```python
from build123d import *

# Parameters (mm, degrees)
F0_R          = 12.7
F1_DEPTH      = 7.874
F3_DEPTH      = 25.4
F3_DEPTH_BACK = 25.4
F5_DEPTH      = 25.4
F5_DEPTH_BACK = 25.4


with BuildPart() as f1:
    # F0 (on Top) → F1 (new body)
    with BuildSketch(Plane.XY):
        Circle(F0_R)
    extrude(amount=F1_DEPTH)

    # F2 (on Front) → F3 (cut, two sides)
    with BuildSketch(Plane.XZ) as f3_sk:
        Polygon((4.5466, 7.874), (-4.5466, 7.874), (-4.3053, 4.1656), (4.3053, 4.1656), align=None)
    extrude(amount=-F3_DEPTH, mode=Mode.SUBTRACT)
    extrude(f3_sk.sketch, amount=F3_DEPTH_BACK, mode=Mode.SUBTRACT)

    # F4 (on Right) → F5 (cut, two sides)
    with BuildSketch(Plane.YZ) as f5_sk:
        Polygon((4.3688, 0), (4.2291, 3.7338), (-4.2291, 3.7338), (-4.3688, 0), align=None)
    extrude(amount=-F5_DEPTH, mode=Mode.SUBTRACT)
    extrude(f5_sk.sketch, amount=F5_DEPTH_BACK, mode=Mode.SUBTRACT)


solid = f1.part
```
Check sheet for the modelled part. Datum: model origin and axes. Units: mm. A direction names the side the tool comes from. Give positions to 0.01 mm unless a question says otherwise; leave off trailing zeros. Order: outer loops, then holes, each group sorted by start corner. A loop starts at its lowest first (then second) coordinate and runs counter-clockwise, first axis right, second up. Notation, with made-up numbers: (17.25, -22) -> (64.25, -22) arc R27 ccw to (64.25, 16) -> close; hole circle Ø11 at (11, 13). An arc over 180 degrees is marked (long way). Use CSV: the item, a comma, the result in double quotes. Start each with the question number.
1) Go/stop test with flat-tipped pins: P1, Ø3, axis at x = 5, y = -8, coming from the -Z side; P2, Ø1, axis at x = -4.5, z = 7, coming from the -Y side; P3, Ø1, axis at x = -7, z = 4, coming from the +Y side; P4, Ø3, axis at x = 2, z = 7, coming from the +Y side. Record where each tip stops, or that it passes through.
2) Set-up check for faces 1 (the face through (0, 0, 4.166)), 2 (the face through (0, 0, 3.734)), 3 (the face through (0, -8, 0)): record each of +Z, -Z, +X, -X, +Y, -Y from which the full face is reachable in a straight line by a thin tool's end or side.
3) Sectioned sample at A-A, the plane x = 0. Record the boundary of the cut face in (y, z).
4) Material ranges on line 1 (Z direction, x = 1.5, y = -5); line 2 (X direction, y = -4.5, z = 5.75); line 3 (Z direction, x = 3.5, y = -3.25), recorded low to high. Write a range as from..to.
5) Sectioned sample at D-D, the plane z = 5. Record the boundary of the cut face in (x, y).
6) Sectioned sample at C-C, the plane z = 2.75. Record the boundary of the cut face in (x, y), plus the area to 3 significant figures.
7) Sectioned sample at B-B, the plane y = 0. Record the boundary of the cut face in (x, z), plus the area to 3 significant figures.
8) Mould release check, pull along X, two halves, no side actions. Record for faces 4 (the face through (-4.428, 0.167, 6.046)), 5 (the face through (0.17, -4.3, 1.89)), 6 (the face through (11.732, -4.864, 3.882)), 7 (the face through (4.424, 0.167, 5.994)): released by +X, released by -X, zero draft, split by the parting line, or undercut.
Recorded:
1,P1,"z = 0"
1,P2,"y = -11.89"
1,P3,"y = 10.91"
1,P4,"through"
2,face 1,"+Z, +Y, -Y"
2,face 2,"-Z, +X, -X"
2,face 3,"-Z, +X, -X, +Y, -Y"
3,outline,"(-12.7, 0) -> (-4.37, 0) -> (-4.23, 3.73) -> (4.23, 3.73) -> (4.37, 0) -> (12.7, 0) -> (12.7, 4.17) -> (-12.7, 4.17) -> close"
4,line 1,"0..4.17"
4,line 2,"-11.88..-4.41, 4.41..11.88"
4,line 3,"3.73..4.17"
5,outline,"(-4.36, -11.93) -> (-4.36, 11.93) arc R12.7 ccw to start; (4.36, -11.93) arc R12.7 ccw to (4.36, 11.93) -> close"
6,outline,"(-11.96, -4.27) arc R12.7 ccw to (11.96, -4.27) -> close; (-11.96, 4.27) -> (11.96, 4.27) arc R12.7 ccw to start"
6,area,"294 mm2"
7,outline,"(-12.7, 3.73) -> (12.7, 3.73) -> (12.7, 7.87) -> (4.55, 7.87) -> (4.31, 4.17) -> (-4.31, 4.17) -> (-4.55, 7.87) -> (-12.7, 7.87) -> close"
7,area,"72.3 mm2"
8,face 4,"undercut"
8,face 5,"zero draft"
8,face 6,"split by the parting line"
8,face 7,"undercut"
